Verification items for this drawing (mm, ordinates from the low corner). A direction names the side the tool comes from. Round coordinates to 2 decimals unless told otherwise and drop trailing zeros. Order: outer loops, then holes, each group sorted by start corner. A loop starts at its lowest first (then second) coordinate and runs counter-clockwise, first axis right, second up.
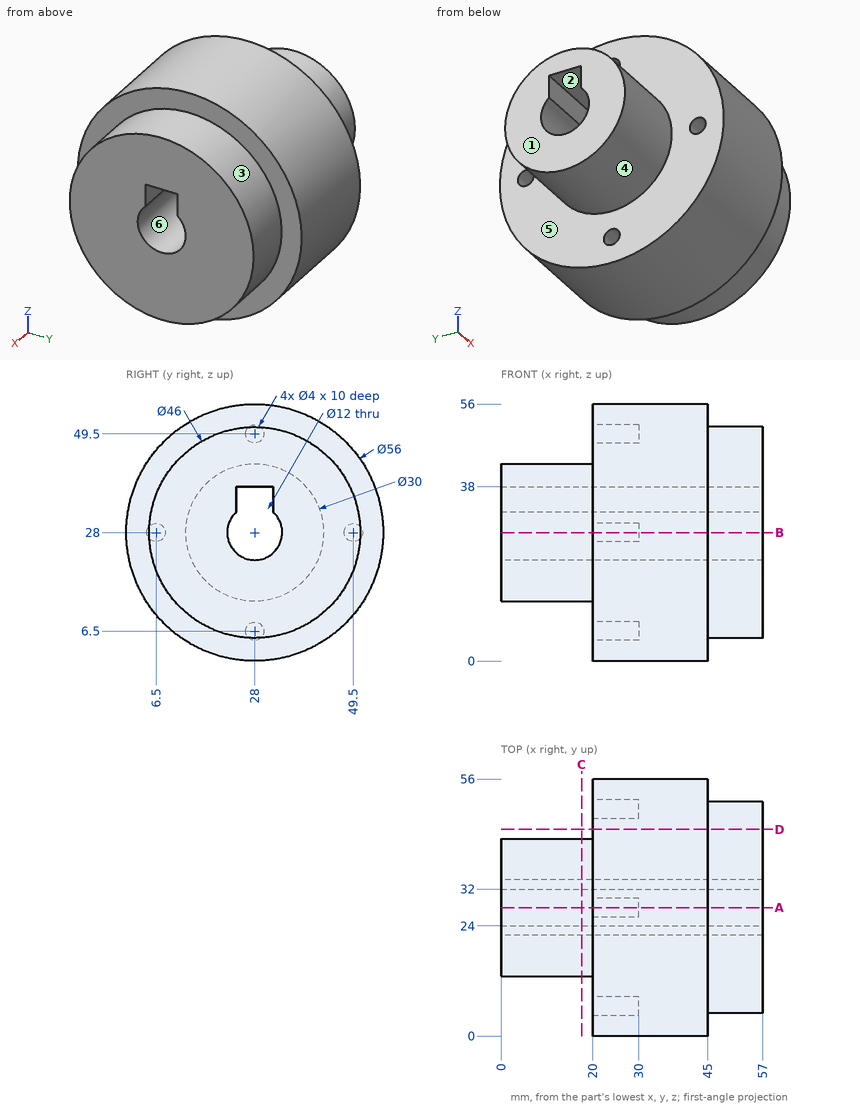
Item 1: Access from +Z, -Z, +X, -X, +Y, -Y to the whole of each face (thin tool, end or side, straight path). Record for the marked faces 1, 2 and 3.
Answer:
face 1: +Z, -Z, -X, +Y, -Y
face 2: +X, -X
face 3: +X
Item 2: Go/stop test with flat-tipped pins: P1, Ø3, axis at y = 48.5, z = 38, coming from the -X side; P2, Ø12, axis at x = 28, z = 46.5, coming from the -Y side (3 decimals); P3, Ø3, axis at x = 15.5, z = 34.5, coming from the -Y side; P4, Ø11, axis at y = 28, z = 28, coming from the -X side. Record where each tip stops, or that it passes through.
Answer:
P1: stops at x = 20
P2: stops at y = 2.945
P3: stops at y = 13.86
P4: passes through
Item 3: Release check for a two-part mould opening along Z. For the marked faces 4, 5 and 6 record: released by +Z, released by -Z, zero draft, split by the parting line, or undercut.
Answer:
face 4: split by the parting line
face 5: zero draft
face 6: undercut
Item 4: Scan lines: line 1 along Z through (x, y) = (25.5, 28); line 2 along Z through (x, y) = (44.5, 28); line 3 along Y through (x, z) = (6.5, 25.5). Record each from-to range of solid material in increasing order.
Answer:
line 1: z = 0 to 4.5, 8.5 to 22, 38 to 47.5, 51.5 to 56
line 2: z = 0 to 22, 38 to 56
line 3: y = 13.21 to 22.55, 33.45 to 42.79
Item 5: Sectioned sample at D-D (y = 45). Record the cut outline in (x, z).
Answer:
outline: (20, 5.75) - (45, 5.75) - (45, 12.51) - (57, 12.51) - (57, 43.49) - (45, 43.49) - (45, 50.25) - (20, 50.25) - close
Item 6: Sectioned sample at A-A (y = 28). Record the cut outline in (x, z).
Answer:
outline: (0, 13) - (20, 13) - (20, 8.5) - (30, 8.5) - (30, 4.5) - (20, 4.5) - (20, 0) - (45, 0) - (45, 5) - (57, 5) - (57, 22) - (0, 22) - close; (0, 38) - (57, 38) - (57, 51) - (45, 51) - (45, 56) - (20, 56) - (20, 51.5) - (30, 51.5) - (30, 47.5) - (20, 47.5) - (20, 43) - (0, 43) - close
Item 7: Sectioned sample at C-C (x = 17.5). Record the cut outline in (y, z), and give its area (3 significant figures).
Answer:
outline: circle Ø30 at (28, 28); hole (24, 32.47) arc R6 ccw (long way) to (32, 32.47) - (32, 38) - (24, 38) - close
area: 558 mm2
Item 8: Sectioned sample at B-B (z = 28). Record the cut outline in (x, y), and give its area (3 significant figures).
Answer:
outline: (0, 13) - (20, 13) - (20, 8.5) - (30, 8.5) - (30, 4.5) - (20, 4.5) - (20, 0) - (45, 0) - (45, 5) - (57, 5) - (57, 22) - (0, 22) - close; (0, 34) - (57, 34) - (57, 51) - (45, 51) - (45, 56) - (20, 56) - (20, 51.5) - (30, 51.5) - (30, 47.5) - (20, 47.5) - (20, 43) - (0, 43) - close
area: 1,790 mm2
